```python
from build123d import *

# Parameters (mm, degrees)
SKETCH1_W           = 25.4
SKETCH1_H           = 50.8
SKETCH1_W_2         = 20.32
SKETCH1_H_2         = 45.72
EXTRUDE_THIN1_DEPTH = 401.6375
SKETCH2_R           = 14.2875
CUT_EXTRUDE1_DEPTH  = 26.4
SKETCH3_R           = 3.175
CUT_EXTRUDE2_DEPTH  = 26.4
SKETCH5_R           = 2.4765
CUT_EXTRUDE4_DEPTH  = 3.81
SKETCH7_R           = 2.4765
CUT_EXTRUDE5_DEPTH  = 51.8
SKETCH8_R           = 2.476504233
CUT_EXTRUDE6_DEPTH  = 3.81


with BuildPart() as part:
    # Sketch1 → Extrude-Thin1 (new body, symmetric)
    with BuildSketch(Plane.XY):
        Rectangle(SKETCH1_W, SKETCH1_H)
        Rectangle(SKETCH1_W_2, SKETCH1_H_2, mode=Mode.SUBTRACT)
    extrude(amount=EXTRUDE_THIN1_DEPTH, both=True)

    # Sketch2 → Cut-Extrude1 (cut, through all)
    with BuildSketch(Plane.ZY.offset(12.7)):
        with Locations((-349.59481695, 0)):
            Circle(SKETCH2_R)
    extrude(amount=-CUT_EXTRUDE1_DEPTH, mode=Mode.SUBTRACT)

    # Sketch3 → Cut-Extrude2 (cut, through all)
    with BuildSketch(Plane.ZY.offset(12.7)):
        with Locations((363.5375, 0)):
            Circle(SKETCH3_R)
        with Locations((287.3375, 0)):
            Circle(SKETCH3_R)
    extrude(amount=-CUT_EXTRUDE2_DEPTH, mode=Mode.SUBTRACT)

    # Sketch5 → Cut-Extrude4 (cut)
    with BuildSketch(Plane.XZ.offset(25.4)):
        with Locations((-5.11e-06, 228.865824925)):
            Circle(SKETCH5_R)
        with Locations((0, 152.665824925)):
            Circle(SKETCH5_R)
    extrude(amount=-CUT_EXTRUDE4_DEPTH, mode=Mode.SUBTRACT)

    # Sketch7 → Cut-Extrude5 (cut, through all)
    with BuildSketch(Plane(origin=(0, 25.4, 0), x_dir=(1, 0, 0), z_dir=(0, 1, 0))):
        with Locations((0, -338.1375)):
            Circle(SKETCH7_R)
        with Locations((0, -363.5375)):
            Circle(SKETCH7_R)
        with Locations((0, -388.9375)):
            Circle(SKETCH7_R)
    extrude(amount=-CUT_EXTRUDE5_DEPTH, mode=Mode.SUBTRACT)

    # Sketch8 → Cut-Extrude6 (cut)
    with BuildSketch(Plane.XZ.offset(25.4)):
        with Locations((-5.001306037, -196.8119)):
            Circle(SKETCH8_R)
        with Locations((-5.048266279, -184.111986821)):
            Circle(SKETCH8_R)
    extrude(amount=-CUT_EXTRUDE6_DEPTH, mode=Mode.SUBTRACT)


solid = part.part
```
CAD build for the part. Positions are in the model's coordinates, mm. A direction names the side the tool comes from. Round coordinates to 2 decimals unless told otherwise and drop trailing zeros. Order: outer loops, then holes, each group sorted by start corner. A loop starts at its lowest first (then second) coordinate and runs counter-clockwise, first axis right, second up. Notation, with made-up numbers: (-31, 10) -> (-14, 10) arc R31 ccw to (-14, 45) -> close; hole circle Ø10 at (74, 38.5). An arc over 180 degrees is marked (long way). One line per question, with ' | ' between items.
Q1. Drop a flat-ended pin along its axis: pin 1 (5.5 mm diameter, centred on y = 0, z = 363.54, fed in from +X). Give the stop position or say it passes through.
Completed:
pin 1: passes through
Q2. Which spindle directions (+Z, -Z, +X, -X, +Y, -Y) get a long thin tool onto all of the face, cutting with end or side? Do faces 5 (the cylindrical face through (-11.448, 9.656, -360.125)), 6 (the flat face through (10.16, 0, 6)). Say none if no direction does.
Completed:
face 5: +X, -X | face 6: +Z, -Z
Q3. Probe probe 1 along Z at (x, y) = (0, -23.45); probe 2 along Y at (x, z) = (-6, -63.5); probe 3 along X at (y, z) = (7, 41). List the from-to ranges inside material, lowest first.
Completed:
probe 1: z = -401.64 to 150.19, 155.14 to 226.39, 231.34 to 335.66, 340.61 to 361.06, 366.01 to 386.46, 391.41 to 401.64 | probe 2: y = -25.4 to -22.86, 22.86 to 25.4 | probe 3: x = -12.7 to -10.16, 10.16 to 12.7
Q4. Two-plate mould, pull along Z, no slides. Class faces 1 (the flat face through (-10.4, 2, 401.638)), 2 (the flat face through (-10.4, 2, -401.638)), 3 (the cylindrical face through (11.412, 9.656, -360.125)), 4 (the flat face through (0, -22.86, 6)): released by +Z, released by -Z, zero draft, split by the parting line, or undercut.
Completed:
face 1: released by +Z | face 2: released by -Z | face 3: undercut | face 4: zero draft
Q5. Slice it at A-A (z = -104.5). Write the cut outline in (x, y).
Completed:
outline: (-12.7, -25.4) -> (12.7, -25.4) -> (12.7, 25.4) -> (-12.7, 25.4) -> close; hole (-10.16, -22.86) -> (10.16, -22.86) -> (10.16, 22.86) -> (-10.16, 22.86) -> close
